Build history of the part. All positions in model axes, mm. A direction names the side the tool comes from. Round coordinates to 2 decimals unless told otherwise and drop trailing zeros. Order: outer loops, then holes, each group sorted by start corner. A loop starts at its lowest first (then second) coordinate and runs counter-clockwise, first axis right, second up. Notation, with made-up numbers: (7.25, 52) -> (55.25, 52) arc R11 cw to (55.25, 61) -> close; hole circle Ø10 at (65, -39.5). An arc over 180 degrees is marked (long way). Answer as a JSON object with one key per item and string values.
Autodesk Inventor part; units mm, degrees
ref_plane "YZ Plane" through (0, 0, 0) normal (1, 0, 0) x (0, 1, 0)
ref_plane "XZ Plane" through (0, 0, 0) normal (0, 1, 0) x (-1, 0, 0)
ref_plane "XY Plane" through (0, 0, 0) normal (0, 0, 1) x (1, 0, 0)
sketch "Sketch1" plane through (0, 0, 0) normal (0, 1, 0) x (-1, 0, 0)
  line L0 (0, -6.685) -> (0, 6.685)
  line L1 (0, -4.775) -> (0, 4.775)
  line L2 (0, -4.775) -> (0.95, -4.775)
  line L3 (0.95, -4.775) -> (0.95, 3.225)
  line L4 (0.95, 3.225) -> (1.875, 3.225)
  line L5 (1.875, 3.225) -> (1.875, 4.775)
  line L6 (2.25, 0) -> (-0.375, 0)
  line L7 (0, 4.775) -> (1.875, 4.775)
  point P0 (0, 0)
  dimension "d0" = 8
  dimension "d1" = 1.9
  dimension "d3" = 3.75
  dimension "d4" = 1.55
revolve "Revolution1" add sketch "Sketch1" angle 360 about axis through (0, 0, -10) along (0, 0, 1)
thread "Thread2"
fillet "Fillet1" radius 0.2 2 edges at (1.875, 0, 4.775) (1.875, 0, 3.225)
sketch "Sketch3" plane through (0, 0, 4.775) normal (0, 0, 1) x (1, 0, 0)
  circle A0 centre (0, 0) radius 1.875
  circle A1 centre (0, 0) radius 1.875
  line L0 (-2.5, -0.325) -> (2.5, -0.325)
  line L1 (2.5, -0.325) -> (2.5, 0.325)
  line L2 (2.5, 0.325) -> (-2.5, 0.325)
  line L3 (-2.5, 0.325) -> (-2.5, -0.325)
  line L4 (-2.5, -0.325) -> (2.5, 0.325) construction
  line L5 (2.5, -0.325) -> (-2.5, 0.325) construction
  dimension "d15" = 0.65
  dimension "d16" = 5
extrude "Extrusion2" cut sketch "Sketch3" against normal blind 0.6 contours A0 L0 L2 | A0 L2 L1 L0 | A0 L0 L3 L2
properties part number "empty"
1) Probe L1, parallel to Z at x = -0.55, y = -0.05 (3 decimals); L2, parallel to Z at x = -1.4, y = -0.65 (3 decimals); L3, parallel to X at y = 0.45, z = 1.5. List the from-to ranges inside material, lowest first. Write a range as from..to.
Checked values:
{"L1": "z = -4.775..4.175", "L2": "z = 3.225..4.775", "L3": "x = -0.84..0.84"}
2) Flat gauge pins, fed straight in: pin 1 Ø2 at (x, y) = (0.5, -1.5) entering from -Z (3 decimals); pin 2 Ø0.7 at (x, z) = (1, 4.5) entering from -Y; pin 3 Ø1 at (y, z) = (0, 0) entering from +X; pin 4 Ø1.5 at (x, z) = (0.5, 0) entering from +Y. Where does each tip first touch, or does it go through?
Checked values:
{"pin 1": "stops at z = -4.775", "pin 2": "stops at y = -1.76", "pin 3": "stops at x = 0.95", "pin 4": "stops at y = 0.95"}
3) Which spindle directions (+Z, -Z, +X, -X, +Y, -Y) get a long thin tool onto all of the face, cutting with end or side? Do faces 1 (the face through (0, 0, -4.775)), 2 (the face through (-1, 1, 3.225)). Say none if no direction does.
Checked values:
{"face 1": "-Z, +X, -X, +Y, -Y", "face 2": "-Z"}
4) Cut at A-A, the plane x = 0. Give the cut face in (y, z) (3 decimals), plus the area to 3 significant figures.
Checked values:
{"outline": "(-1.875, 3.425) arc R0.2 ccw to (-1.675, 3.225) -> (-0.95, 3.225) -> (-0.95, -4.775) -> (0.95, -4.775) -> (0.95, 3.225) -> (1.675, 3.225) arc R0.2 ccw to (1.875, 3.425) -> (1.875, 4.575) arc R0.2 ccw to (1.675, 4.775) -> (0.325, 4.775) -> (0.325, 4.175) -> (-0.325, 4.175) -> (-0.325, 4.775) -> (-1.675, 4.775) arc R0.2 ccw to (-1.875, 4.575) -> close", "area": "20.6 mm²"}
5) Cut at B-B, the plane y = 0. Give the cut face in (x, z) (3 decimals), plus the area to 3 significant figures.
Checked values:
{"outline": "(-1.875, 3.425) arc R0.2 ccw to (-1.675, 3.225) -> (-0.95, 3.225) -> (-0.95, -4.775) -> (0.95, -4.775) -> (0.95, 3.225) -> (1.675, 3.225) arc R0.2 ccw to (1.875, 3.425) -> (1.875, 4.175) -> (-1.875, 4.175) -> close", "area": "18.7 mm²"}
6) Cut at C-C, the plane z = -1.75. Give the cut face in (x, y).
Checked values:
{"outline": "circle Ø1.9 at (0, 0)"}
7) Cut at D-D, the plane z = 4. Give the cut face in (x, y) (3 decimals).
Checked values:
{"outline": "circle Ø3.75 at (0, 0)"}
